Geometry: see drawing. Coordinates: mm, zero at the bounding-box minimum. A direction names the side the tool comes from. Round coordinates to 2 decimals unless told otherwise and drop trailing zeros. Loops run counter-clockwise (first coordinate to the right, second up) from the corner with the lowest first, then second, coordinate; pieces in that order, holes last.
(1) Section C-C, the plane x = 30. Return the cut outline in (y, z), plus the area to 3 significant figures.
(2) First-contact query: pin 1 Ø6.5 at (x, z) = (50, 84) entering from +Y; pin 2 Ø1.7 at (x, y) = (50.5, 12) entering from +Z; pin 3 Ø4.5 at (x, y) = (13.5, 13) entering from +Z. Flat tips, straight axial feed; report the tip coordinate or a pass-through.
(3) Set-up query: the marked faces 1 and 2. Return all of +Z, -Z, +X, -X, +Y, -Y with unobstructed straight access to the full face (end or side cutting, diameter ignored); none if empty.
(4) Section B-B, the plane y = 2.5. Return the cut outline in (x, z).
(5) Section D-D, the plane y = 12. Return the cut outline in (x, z).
(6) Material intervals for probe 1 along X at (y, z) = (5.25, 84); probe 2 along Z at (x, y) = (6, 4.5); probe 3 along Z at (x, y) = (30, 5.25), sorted ascending.
(7) Section A-A, the plane z = 84. Return the cut outline in (x, y), plus the area to 3 significant figures.
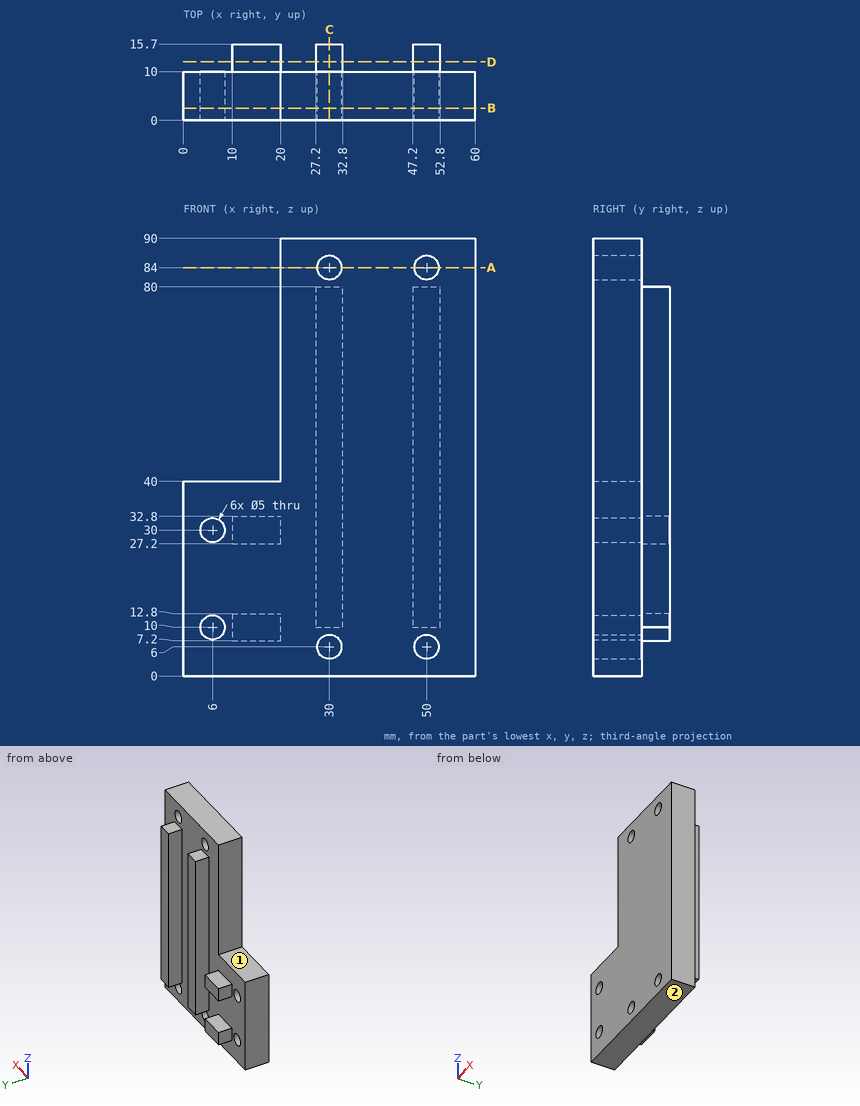
Output values:
1. outline: (0, 0) - (10, 0) - (10, 3.5) - (0, 3.5) - close; (0, 8.5) - (10, 8.5) - (10, 10) - (15.7, 10) - (15.7, 80) - (10, 80) - (10, 81.5) - (0, 81.5) - close; (0, 86.5) - (10, 86.5) - (10, 90) - (0, 90) - close
1. area: 1,200 mm2
2. pin 1: stops at y = 10
2. pin 2: stops at z = 80
2. pin 3: stops at z = 32.8
3. face 1: +Z, -X, +Y, -Y
3. face 2: -Z, +X, -X, +Y, -Y
4. outline: (0, 0) - (60, 0) - (60, 90) - (20, 90) - (20, 40) - (0, 40) - close; hole circle Ø5 at (6, 10); hole circle Ø5 at (6, 30); hole circle Ø5 at (30, 6); hole circle Ø5 at (30, 84); hole circle Ø5 at (50, 6); hole circle Ø5 at (50, 84)
5. outline: (10, 7.2) - (20, 7.2) - (20, 12.8) - (10, 12.8) - close; (10, 27.2) - (20, 27.2) - (20, 32.8) - (10, 32.8) - close; (27.2, 10) - (32.8, 10) - (32.8, 80) - (27.2, 80) - close; (47.2, 10) - (52.8, 10) - (52.8, 80) - (47.2, 80) - close
6. probe 1: x = 20 to 27.5, 32.5 to 47.5, 52.5 to 60
6. probe 2: z = 0 to 7.5, 12.5 to 27.5, 32.5 to 40
6. probe 3: z = 0 to 3.5, 8.5 to 81.5, 86.5 to 90
7. outline: (20, 0) - (27.5, 0) - (27.5, 10) - (20, 10) - close; (32.5, 0) - (47.5, 0) - (47.5, 10) - (32.5, 10) - close; (52.5, 0) - (60, 0) - (60, 10) - (52.5, 10) - close
7. area: 300 mm2
